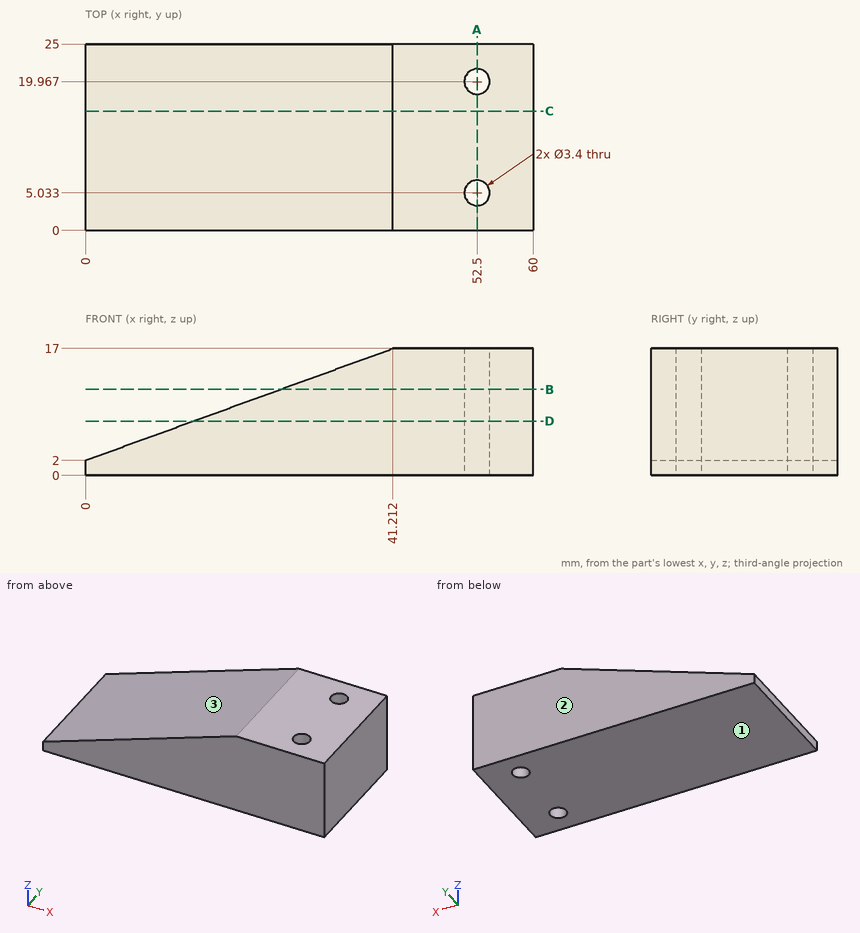
Design review of the part shown in the three views and the two pictorial views. Dimensions are in mm from the part's minimum x, y and z. Coordinates: 2 decimals unless noted, no trailing zeros. Order: outer loops, then holes, each group sorted by start corner. A loop starts at its lowest first (then second) coordinate and runs counter-clockwise, first axis right, second up.
Item 1: For line 1 (Y direction, x = 52.5, z = 4.5); line 2 (Y direction, x = 51, z = 11.75) (1 decimal); line 3 (Z direction, x = 27, y = 5), list the stretches that pass through material, from the lowest coordinate up.
Item 2: Take a section at C-C, the plane y = 16. Write out the cut boundary in (x, z).
Item 3: Take a section at D-D, the plane z = 7.25. Write out the cut boundary in (x, y).
Item 4: The part is to be moulded in two halves that separate along Z. For the marked faces 1, 2 and 3, say which applies: pulls with the +Z half, pulls with the -Z half, needs draft (parallel to the pull), parting line crosses it, or undercut.
Item 5: For pin 1 Ø2.5 at (x, y) = (52.5, 19.97) entering from -Z, flat-tipped, find the tip position at first contact; note if it passes through.
Item 6: Take a section at A-A, the plane x = 52.5. Write out the cut boundary in (y, z).
Item 7: Take a section at B-B, the plane z = 11.5. Write out the cut boundary in (x, y), then the cut area to 3 significant figures.
The answers:
1. line 1: y = 0 to 3.33, 6.73 to 18.27, 21.67 to 25
1. line 2: y = 0 to 4.2, 5.8 to 19.2, 20.8 to 25
1. line 3: z = 0 to 11.83
2. outline: (0, 0) - (60, 0) - (60, 17) - (41.21, 17) - (0, 2) - close
3. outline: (14.42, 0) - (60, 0) - (60, 25) - (14.42, 25) - close; hole circle Ø3.4 at (52.5, 5.03); hole circle Ø3.4 at (52.5, 19.97)
4. face 1: pulls with the -Z half
4. face 2: needs draft
4. face 3: pulls with the +Z half
5. pin 1: passes through
6. outline: (0, 0) - (3.33, 0) - (3.33, 17) - (0, 17) - close; (6.73, 0) - (18.27, 0) - (18.27, 17) - (6.73, 17) - close; (21.67, 0) - (25, 0) - (25, 17) - (21.67, 17) - close
7. outline: (26.1, 0) - (60, 0) - (60, 25) - (26.1, 25) - close; hole circle Ø3.4 at (52.5, 5.03); hole circle Ø3.4 at (52.5, 19.97)
7. area: 829 mm2
